Verification items for the finished model (mm, model axes). Face numbers are marked on the shaded views. A direction names the side the tool comes from. Round coordinates to 2 decimals unless told otherwise and drop trailing zeros. Write each loop counter-clockwise with the first axis right and the second up, starting at its lowest first coordinate (ties: lowest second). Pieces come first, ordered by that corner, then holes. Notation, with made-up numbers: (59, 3) - (98, 3) arc R23 cw to (98, 26) - close; hole circle Ø2 at (61.25, 46). An arc over 180 degrees is marked (long way). Answer as a JSON object with one key per item and string values. Group by question number.
1) Set-up check for the marked faces 5 and 6: record each of +Z, -Z, +X, -X, +Y, -Y from which the full face is reachable in a straight line by a thin tool's end or side.
2) Go/stop test with flat-tipped pins: pin 1 Ø1.9 at (x, z) = (16.5, 0) entering from -Y; pin 2 Ø3 at (y, z) = (7.5, 3) entering from +X. Record where each tip stops, or that it passes through.
3) Mould release check, pull along Z, two halves, no side actions. Record for the marked faces 1, 2, 3 and 4: +Z half, -Z half, draft (parallel to the pull), parting line (faces both ways), or undercut.
4) Section check C-C (y = 2.25). Enter the section's corners in (x, z), then the cut area to 3 significant figures.
5) Section check A-A (z = 0). Enter the section's corners in (x, y).
6) Section check B-B (x = 0). Enter the section's corners in (y, z).
7) Section check D-D (y = 10.75). Enter the section's corners in (x, z).
8) Thickness scan on line 1 (Z direction, x = 0, y = 1.55); line 2 (Y direction, x = -11, z = -8); line 3 (Z direction, x = 4, y = 2.5). Record the ranges inside material, lowest first.
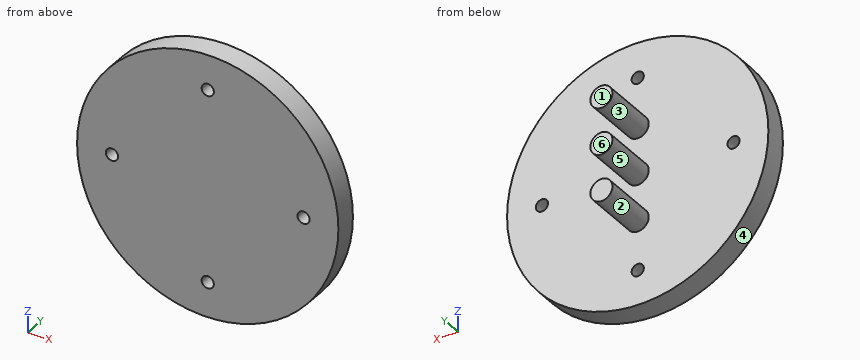
Autodesk Inventor part; units mm, degrees
ref_plane "YZ Plane" through (0, 0, 0) normal (1, 0, 0) x (0, 1, 0)
ref_plane "XZ Plane" through (0, 0, 0) normal (0, 1, 0) x (-1, 0, 0)
ref_plane "XY Plane" through (0, 0, 0) normal (0, 0, 1) x (1, 0, 0)
sketch "Sketch1" plane through (0, 0, 0) normal (0, 1, 0) x (-1, 0, 0)
  circle A0 centre (0, 0) radius 22.5
  dimension "d0" = 45
extrude "Extrusion1" add sketch "Sketch1" along normal blind 4
sketch "Sketch2" plane through (0, 4, 0) normal (0, 1, 0) x (1, 0, 0)
  line L0 (0, 0) -> (0, 8) construction
  line L1 (0, 0) -> (0, -8) construction
  circle A0 centre (0, 8) radius 1.9
  circle A1 centre (0, 0) radius 1.9
  circle A2 centre (0, -8) radius 1.9
  dimension "d3" = 8
  dimension "d4" = 8
  dimension "d5" = 3.8
  dimension "d6" = 3.8
  dimension "d7" = 3.8
extrude "Extrusion2" add sketch "Sketch2" along normal blind 10
sketch "Sketch7" plane through (0, 0, 0) normal (0, -1, 0) x (1, 0, 0)
  circle A0 centre (0, 0) radius 16.5 construction
  circle A1 centre (0, 16.5) radius 1.05
  circle A2 centre (16.5, 0) radius 1.05
  circle A3 centre (-16.5, 0) radius 1.05
  circle A4 centre (0, -16.5) radius 1.05
  dimension "d42" = 33
  dimension "d43" = 2.1
  dimension "d44" = 2.1
  dimension "d45" = 2.1
  dimension "d46" = 2.1
extrude "Extrusion6" cut sketch "Sketch7" against normal blind 5
properties part number "Motor Mount Barebones bigscrew4mmheight"
Returned:
{
 "1": {"face 5": "+Y", "face 6": "+Z, -Z, +X, -X, +Y"},
 "2": {"pin 1": "through", "pin 2": "x = 1.17"},
 "3": {"face 1": "draft", "face 2": "undercut", "face 3": "undercut", "face 4": "parting line"},
 "4": {"outline": "circle Ø45 at (0, 0); hole circle Ø2.1 at (-16.5, 0); hole circle Ø2.1 at (0, -16.5); hole circle Ø2.1 at (0, 16.5); hole circle Ø2.1 at (16.5, 0)", "area": "1,580 mm2"},
 "5": {"outline": "(-22.5, 0) - (-17.55, 0) - (-17.55, 4) - (-22.5, 4) - close; (-15.45, 0) - (15.45, 0) - (15.45, 4) - (1.9, 4) - (1.9, 14) - (-1.9, 14) - (-1.9, 4) - (-15.45, 4) - close; (17.55, 0) - (22.5, 0) - (22.5, 4) - (17.55, 4) - close"},
 "6": {"outline": "(0, -22.5) - (4, -22.5) - (4, -17.55) - (0, -17.55) - close; (0, -15.45) - (4, -15.45) - (4, -9.9) - (14, -9.9) - (14, -6.1) - (4, -6.1) - (4, -1.9) - (14, -1.9) - (14, 1.9) - (4, 1.9) - (4, 6.1) - (14, 6.1) - (14, 9.9) - (4, 9.9) - (4, 15.45) - (0, 15.45) - close; (0, 17.55) - (4, 17.55) - (4, 22.5) - (0, 22.5) - close"},
 "7": {"outline": "circle Ø3.8 at (0, -8); circle Ø3.8 at (0, 0); circle Ø3.8 at (0, 8)"},
 "8": {"line 1": "-22.5 to -17.55, -15.45 to 15.45, 17.55 to 22.5", "line 2": "0 to 4", "line 3": "-22.14 to 22.14"}
}
